Autodesk Inventor part; units mm, degrees
ref_plane "YZ Plane" through (0, 0, 0) normal (1, 0, 0) x (0, 1, 0)
ref_plane "XZ Plane" through (0, 0, 0) normal (0, 1, 0) x (-1, 0, 0)
ref_plane "XY Plane" through (0, 0, 0) normal (0, 0, 1) x (1, 0, 0)
sketch "Sketch1" plane through (0, 0, 0) normal (0, 0, 1) x (1, 0, 0)
  circle A0 centre (0, 0) radius 28.575
  line L0 (0, 7.3323) -> (6.35, 3.6662)
  line L1 (6.35, 3.6662) -> (6.35, -3.6662)
  line L2 (6.35, -3.6662) -> (0, -7.3323)
  line L3 (0, -7.3323) -> (-6.35, -3.6662)
  line L4 (-6.35, -3.6662) -> (-6.35, 3.6662)
  line L5 (-6.35, 3.6662) -> (0, 7.3323)
  dimension "d0" = 57.15
  dimension "d1" = 12.7
extrude "Extrusion1" add sketch "Sketch1" along normal blind 3.175
sketch "Sketch3" plane through (0, 0, 3.175) normal (0, 0, 1) x (1, 0, 0)
  line L0 (6.35, 3.6662) -> (6.35, -3.6662)
  line L1 (6.35, -3.6662) -> (0, -7.3323)
  line L2 (0, -7.3323) -> (-6.35, -3.6662)
  line L3 (-6.35, -3.6662) -> (-6.35, 3.6662)
  line L4 (-6.35, 3.6662) -> (0, 7.3323)
  line L5 (0, 7.3323) -> (6.35, 3.6662)
  circle A0 centre (0, 0) radius 28.575
  circle A1 centre (0, 0) radius 22.225
  dimension "d8" = 44.45
extrude "Extrusion3" add sketch "Sketch3" along normal blind 6.35 contours A1
properties part number "Tube End Cap"
CAD build for the part. Positions are in the model's coordinates, mm. A direction names the side the tool comes from. Round coordinates to 2 decimals unless told otherwise and drop trailing zeros. Order: outer loops, then holes, each group sorted by start corner. A loop starts at its lowest first (then second) coordinate and runs counter-clockwise, first axis right, second up.
Q1. Two-plate mould, pull along Y, no slides. Class faces 1 (the flat face through (-3.219, 5.474, 4.696)), 2 (the flat face through (3.131, 5.525, 4.696)), 3 (the cylindrical face through (21.199, -6.676, 6.306)), 4 (the flat face through (-7, 0, 0)): pulls with the +Y half, pulls with the -Y half, needs draft (parallel to the pull), parting line crosses it, or undercut.
Q2. Drop flat-ended pins along their axis: pin 1 (1 mm diameter, centred on x = -4.5, z = 6.5, fed in from -Y); pin 2 (1.5 mm diameter, centred on x = -7, z = 8.5, fed in from +Y); pin 3 (1.5 mm diameter, centred on x = 20, z = 3.5, fed in from -Y). Give the stop position or say it passes through.
Q3. Which spindle directions (+Z, -Z, +X, -X, +Y, -Y) get a long thin tool onto all of the face, cutting with end or side? Do faces 5 (the flat face through (-6.35, 0, 5)), 6 (the flat face through (15, -17, 3.175)), 7 (the flat face through (-5, -5, 9.525)). Say none if no direction does.
Q4. Wall check: L1, parallel to Z at x = 15, y = 17.5 (3 decimals); L2, parallel to Y at x = 3, z = 6.75; L3, parallel to Y at x = -2, z = 3.5. Give the ranges that are in metal, low to high.
Q5. Slice it at C-C (x = 15.5). Write the cut outline in (y, z) (3 decimals).
Q6. Slice it at A-A (y = 0). Write the cut outline in (x, z) (3 decimals), and give its area (3 significant figures).
Q7. Slice it at D-D (y = 15). Write the cut outline in (x, z) (3 decimals), and give its area (3 significant figures).
Q8. Slice it at B-B (z = 4.5). Write the cut outline in (x, y) (3 decimals), and give its area (3 significant figures).
Results below:
1. face 1: undercut
1. face 2: undercut
1. face 3: parting line crosses it
1. face 4: needs draft
2. pin 1: stops at y = -21.86
2. pin 2: stops at y = 21.33
2. pin 3: stops at y = -21.05
3. face 5: +Z, -Z
3. face 6: +Z
3. face 7: +Z, +X, -X, +Y, -Y
4. L1: z = 0 to 3.175
4. L2: y = -22.02 to -5.6, 5.6 to 22.02
4. L3: y = -22.13 to -6.18, 6.18 to 22.13
5. outline: (-24.006, 0) - (24.006, 0) - (24.006, 3.175) - (15.928, 3.175) - (15.928, 9.525) - (-15.928, 9.525) - (-15.928, 3.175) - (-24.006, 3.175) - close
6. outline: (-28.575, 0) - (-6.35, 0) - (-6.35, 9.525) - (-22.225, 9.525) - (-22.225, 3.175) - (-28.575, 3.175) - close; (6.35, 0) - (28.575, 0) - (28.575, 3.175) - (22.225, 3.175) - (22.225, 9.525) - (6.35, 9.525) - close
6. area: 343 mm2
7. outline: (-24.321, 0) - (24.321, 0) - (24.321, 3.175) - (16.4, 3.175) - (16.4, 9.525) - (-16.4, 9.525) - (-16.4, 3.175) - (-24.321, 3.175) - close
7. area: 363 mm2
8. outline: circle Ø44.45 at (0, 0); hole (-6.35, -3.666) - (0, -7.332) - (6.35, -3.666) - (6.35, 3.666) - (0, 7.332) - (-6.35, 3.666) - close
8. area: 1,410 mm2
